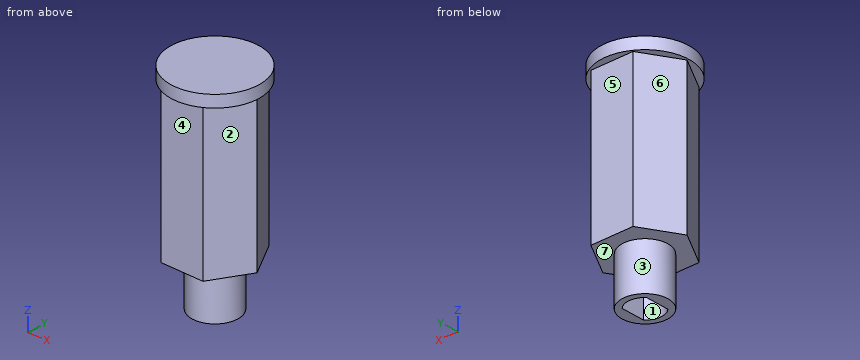
from build123d import *

# Parameters (mm, degrees)
SKETCH1_R           = 3.9
BOSS_EXTRUDE1_DEPTH = 8
BOSS_EXTRUDE2_DEPTH = 25.5
SKETCH3_R           = 7.5
BOSS_EXTRUDE3_DEPTH = 2


with BuildPart() as part:
    # Sketch1 → Boss-Extrude1 (new body)
    with BuildSketch(Plane.XY):
        Circle(SKETCH1_R)
        with BuildLine():
            Line((-2.080769089, -2.02), (-2.080769089, 2.02))
            ThreePointArc((-2.080769089, 2.02), (0, 2.9), (2.080769089, 2.02))
            Line((2.080769089, 2.02), (2.080769089, -2.02))
            ThreePointArc((2.080769089, -2.02), (0, -2.9), (-2.080769089, -2.02))
        make_face(mode=Mode.SUBTRACT)
    extrude(amount=BOSS_EXTRUDE1_DEPTH)

    # Sketch2 → Boss-Extrude2 (add)
    with BuildSketch(Plane.XY.offset(8)):
        Polygon((3.6, 6.235382907), (-3.6, 6.235382907), (-7.2, 0), (-3.6, -6.235382907), (3.6, -6.235382907), (7.2, 0), align=None)
    extrude(amount=BOSS_EXTRUDE2_DEPTH)

    # Sketch3 → Boss-Extrude3 (add)
    with BuildSketch(Plane.XY.offset(33.5)):
        Circle(SKETCH3_R)
    extrude(amount=BOSS_EXTRUDE3_DEPTH)


solid = part.part
CAD build for the part. Positions are in the model's coordinates, mm. Face numbers are marked on the shaded views. A direction names the side the tool comes from. Give positions to 0.01 mm unless a question says otherwise; leave off trailing zeros. Write each loop counter-clockwise with the first axis right and the second up, starting at its lowest first coordinate (ties: lowest second). Pieces come first, ordered by that corner, then holes. Notation, with made-up numbers: M 32.25,-29.5 L 76.25,-29.5 A15 cw 76.25,-5.5 Z; hole C 65.5,72 d9. An arc over 180 degrees is marked long. Put each result on its own line as item: value. Start each with the question number.
(1) Band-saw the part on B-B, the plane y = 1. Write the cut outline in (x, z), and give its area (3 significant figures).
(2) Band-saw the part on D-D, the plane z = 22. Write the cut outline in (x, y).
(3) Mould opens along X. For the marked faces 1, 2, 3 and 4 say: +X half, -X half, draft (parallel to the pull), parting line (faces both ways), or undercut.
(4) Which spindle directions (+Z, -Z, +X, -X, +Y, -Y) get a long thin tool onto all of the face, cutting with end or side? Do the marked faces 5, 6 and 7. Say none if no direction does.
(5) Band-saw the part on C-C, the plane x = 0. Write the cut outline in (y, z), and give its area (3 significant figures).
(6) Probe L1, parallel to X at y = -1.5, z = 4.5; L2, parallel to Z at x = 0.25, y = -1; L3, parallel to Z at x = 6.5, y = -2.75. List the from-to ranges inside material, lowest first.
(7) Band-saw the part on A-A, the plane z = 3.5. Write the cut outline in (x, y), and give its area (3 significant figures).
(8) Flat gauge pins, fed straight in: pin 1 Ø8 at (x, z) = (5, 17.5) entering from +Y; pin 2 Ø1 at (x, y) = (-3.5, -4.5) entering from -Z; pin 3 Ø4 at (x, z) = (-2.5, 8) entering from -Y. Where does each tip first touch, or does it go through?
Response values:
1. outline: M -7.43,33.5 L -6.62,33.5 L -6.62,8 L -3.77,8 L -3.77,0 L -2.08,0 L -2.08,8 L 2.08,8 L 2.08,0 L 3.77,0 L 3.77,8 L 6.62,8 L 6.62,33.5 L 7.43,33.5 L 7.43,35.5 L -7.43,35.5 Z
1. area: 395 mm2
2. outline: M -7.2,0 L -3.6,-6.24 L 3.6,-6.24 L 7.2,0 L 3.6,6.24 L -3.6,6.24 Z
3. face 1: undercut
3. face 2: +X half
3. face 3: parting line
3. face 4: draft
4. face 5: -Z, +X, -X, +Y
4. face 6: -Z, -X, +Y
4. face 7: -Z
5. outline: M -7.5,33.5 L -6.24,33.5 L -6.24,8 L -3.9,8 L -3.9,0 L -2.9,0 L -2.9,8 L 2.9,8 L 2.9,0 L 3.9,0 L 3.9,8 L 6.24,8 L 6.24,33.5 L 7.5,33.5 L 7.5,35.5 L -7.5,35.5 Z
5. area: 364 mm2
6. L1: x = -3.6 to -2.08, 2.08 to 3.6
6. L2: z = 8 to 35.5
6. L3: z = 33.5 to 35.5
7. outline: C 0,0 d7.8; hole M -2.08,-2.02 A2.9 ccw 2.08,-2.02 L 2.08,2.02 A2.9 ccw -2.08,2.02 Z
7. area: 25.9 mm2
8. pin 1: stops at y = 6.24
8. pin 2: stops at z = 8
8. pin 3: stops at y = -6.24
